from build123d import *

# Parameters (mm, degrees)
SKETCH_2_W          = 8
SKETCH_2_H          = 8
EXTRUDE_1_DEPTH     = 8
SKETCH_4_R          = 5
CUT_EXTRUDE_1_DEPTH = 6
FILLET_1_R          = 0.5


with BuildPart() as part:
    # 草图1 → 旋转1 (revolve)
    with BuildSketch(Plane.XY, mode=Mode.PRIVATE) as revolve_1_sk:
        with BuildLine():
            Line((0, 0), (5, 0))
            Line((5, 0), (5, 2))
            Line((5, 2), (4, 2))
            Line((4, 2), (4, 5))
            Line((4, 5), (5, 5))
            Line((5, 5), (5, 7))
            Line((5, 7), (6, 8))
            ThreePointArc((6, 8), (5.451628729, 27.225245427), (3.979757576, 46.401907496))
            ThreePointArc((3.979757576, 46.401907496), (2.682570597, 48.967122342), (0, 50))
            Line((0, 50), (0, 0))
        make_face()
    revolve(revolve_1_sk.sketch.rotate(Axis((0, -56.22118461, 0), (0, 1, 0)), 90), axis=Axis((0, -56.22118461, 0), (0, 1, 0)))

    # 草图2 → 凸台-拉伸1 (add)
    with BuildSketch(Plane.XZ):
        Rectangle(SKETCH_2_W, SKETCH_2_H)
    extrude(amount=EXTRUDE_1_DEPTH)

    # 草图3 → 旋转2 (revolve)
    with BuildSketch(Plane.XY, mode=Mode.PRIVATE) as revolve_2_sk:
        with BuildLine():
            Line((4, -4), (4, -1))
            Line((4, -1), (6, -1))
            Line((6, -1), (6, 1))
            Line((6, 1), (12, 1))
            Line((12, 1), (12, -0.825))
            Line((12, -0.825), (15, -0.825))
            Line((15, -0.825), (15, -1.325))
            Line((15, -1.325), (7, -1.325))
            Line((7, -1.325), (7, -3.6))
            Line((7, -3.6), (12, -3.6))
            ThreePointArc((12, -3.6), (12.282842712, -3.717157288), (12.4, -4))
            Line((12.4, -4), (4, -4))
        make_face()
    revolve(revolve_2_sk.sketch.rotate(Axis((-4, -4, 0), (1, 0, 0)), 90), axis=Axis((-4, -4, 0), (1, 0, 0)))

    # 草图4 → 切除-拉伸1 (cut)
    with BuildSketch(Plane(origin=(12, 0, 0), x_dir=(0, 0, -1), z_dir=(1, 0, 0))):
        with Locations((0, -4)):
            Circle(SKETCH_4_R)
        Polygon((2.309401077, 0), (-2.309401077, 0), (-4.618802154, -4), (-2.309401077, -8), (2.309401077, -8), (4.618802154, -4), align=None, mode=Mode.SUBTRACT)
    extrude(amount=-CUT_EXTRUDE_1_DEPTH, mode=Mode.SUBTRACT)

    # 圆角1
    fillet_1_edges = [part.edges().sort_by_distance(p)[0] for p in [
        (4, -4, -4),
        (4, -4, 4),
        (-4, -4, 4),
        (-4, -4, -4),
        (4, -8, 0),
        (0, -8, 4),
        (-4, -8, 0),
        (0, -8, -4),
        (9, 0, -2.309401077),
        (9, 0, 2.309401077),
        (9, -4, 4.618802154),
        (9, -8, 2.309401077),
        (9, -8, -2.309401077),
        (9, -4, -4.618802154),
    ]]
    fillet(fillet_1_edges, radius=FILLET_1_R)


solid = part.part
Input: part model. Units: mm. Frame: model coordinates. A direction names the side the tool comes from. Round coordinates to 2 decimals unless told otherwise and drop trailing zeros. Order: outer loops, then holes, each group sorted by start corner. A loop starts at its lowest first (then second) coordinate and runs counter-clockwise, first axis right, second up. Notation, with made-up numbers: (41, 42.5) - (85, 42.5) arc R30 cw to (85, 67.5) - close; hole circle Ø7 at (-28, 11.25). An arc over 180 degrees is marked (long way). Use a Markdown table: item, result.
1. Section A-A on x = 10.5. Return the cut outline in (y, z) (3 decimals), then the cut area to 3 significant figures.
Evaluation:
| item | result |
|---|---|
| outline | (-8, -2.021) arc R0.5 ccw to (-7.75, -2.454) - (-4.25, -4.474) arc R0.5 ccw to (-3.75, -4.474) - (-0.25, -2.454) arc R0.5 ccw to (0, -2.021) - (0, 2.021) arc R0.5 ccw to (-0.25, 2.454) - (-3.75, 4.474) arc R0.5 ccw to (-4.25, 4.474) - (-7.75, 2.454) arc R0.5 ccw to (-8, 2.021) - close; circle Ø0.8 at (-4, 0); hole circle Ø5.35 at (-4, 0) |
| area | 33.4 mm^2 |
2. Material intervals for probe 1 along Y at (x, z) = (9, 0) (3 decimals); probe 2 along Y at (x, z) = (13, 0) (3 decimals); probe 3 along X at (y, z) = (-1, 1.25), sorted ascending.
Evaluation:
| item | result |
|---|---|
| probe 1 | -8 to -6.675, -4.4 to -3.6, -1.325 to 0 |
| probe 2 | -7.175 to -6.675, -1.325 to -0.825 |
| probe 3 | -4 to 4, 6 to 12 |
3. Access query for faces 4 (the face through (7, -3, 0)), 5 (the face through (6, -3, -3)), 6 (the face through (3.7, 0, -3.6)). Directions: +Z, -Z, +X, -X, +Y, -Y. A direction counts if a zero-diameter tool reaches every point of the face in a straight line with its end or side. Return the directions, or none.
Evaluation:
| item | result |
|---|---|
| face 4 | +X |
| face 5 | none |
| face 6 | -Z, +X |
4. Mould query, pull axis Z, two halves, no side actions, for faces 1 (the face through (10.94, -1.39, -0.58)), 2 (the face through (0, 1, 5)), 3 (the face through (9, 0, 0)). Classes: +Z half, -Z half, draft (parallel to the pull), parting line (faces both ways), or undercut.
Evaluation:
| item | result |
|---|---|
| face 1 | undercut |
| face 2 | parting line |
| face 3 | draft |
5. Section B-B on x = 13.75. Return the cut outline in (y, z) (3 decimals).
Evaluation:
| item | result |
|---|---|
| outline | circle Ø6.35 at (-4, 0); hole circle Ø5.35 at (-4, 0) |
6. First-contact query: pin 1 (2.5 mm diameter, centred on y = -3.5, z = -1, fed in from +X); pin 2 (2 mm diameter, centred on x = -0.5, z = 0, fed in from +Y); pin 3 (0.5 mm diameter, centred on x = -0.5, z = -4.5, fed in from -Y); pin 4 (5.5 mm diameter, centred on y = -4, z = -1, fed in from -X). Flat tips, straight axial feed; report the tip coordinate or a pass-through.
Evaluation:
| item | result |
|---|---|
| pin 1 | x = 12.4 |
| pin 2 | y = 50 |
| pin 3 | y = 0 |
| pin 4 | x = -4 |
